from build123d import *

# Parameters (mm, degrees)
F0_R            = 304.8
F1_DEPTH        = 25.4
F2_DEPTH        = 25.4
F2_COPIES_COUNT = 31
F3_R            = 296.8625
F3_R_2          = 290.5125
F4_DEPTH        = 2.54
F5_R            = 296.8625
F5_R_2          = 290.5125
F6_DEPTH        = 2.54


# Not quite as in the source:
# - a pattern or mirror of a feature is missing from the dataset's text; its kind, count and spacing are read off the source's solid


with BuildPart() as f1:
    # F0 (on Top) → F1 (new body)
    with BuildSketch(Plane.XY):
        Circle(F0_R)
        with BuildLine():
            ThreePointArc((-139.9074929569, 241.8475830239), (139.5962149699, 242.0273884627), (279.4, 0))
            ThreePointArc((279.4, 0), (8.5793400064, -279.2682490457), (-278.873120437, -17.1505888444))
            Line((-278.873120437, -17.1505888444), (-284.48, -19.05))
            Line((-284.48, -19.05), (-284.48, 19.05))
            Line((-284.48, 19.05), (-278.873120437, 17.1505888444))
            ThreePointArc((-278.873120437, 17.1505888444), (-278.0539903617, 27.392306291), (-276.8588574341, 37.5969820635))
            Line((-276.8588574341, 37.5969820635), (-282.7052908844, 36.7727961626))
            Line((-282.7052908844, 36.7727961626), (-275.2642057328, 74.52500298))
            Line((-275.2642057328, 74.52500298), (-270.0959710932, 71.5019328355))
            ThreePointArc((-270.0959710932, 71.5019328355), (-267.303871456, 81.3203560288), (-264.1549850662, 91.0302359916))
            Line((-264.1549850662, 91.0302359916), (-270.1311147854, 91.3975495928))
            Line((-270.1311147854, 91.3975495928), (-255.2871620754, 126.8976403584))
            Line((-255.2871620754, 126.8976403584), (-250.8902083052, 122.9571607373))
            ThreePointArc((-250.8902083052, 122.9571607373), (-246.2317976323, 132.0388648646), (-241.2447866782, 140.9443610102))
            Line((-241.2447866782, 140.9443610102), (-247.0326592074, 142.4729997596))
            Line((-247.0326592074, 142.4729997596), (-225.5328396666, 174.384889715))
            Line((-225.5328396666, 174.384889715), (-221.9907783353, 169.6598194449))
            ThreePointArc((-221.9907783353, 169.6598194449), (-215.6401479473, 177.6617195494), (-209.0012374477, 185.4261112825))
            Line((-209.0012374477, 185.4261112825), (-214.453995901, 188.1291797331))
            Line((-214.453995901, 188.1291797331), (-187.0092810122, 215.058314286))
            Line((-187.0092810122, 215.058314286), (-184.5245635336, 209.7976297595))
            ThreePointArc((-184.5245635336, 209.7976297595), (-176.734130204, 216.4010333179), (-168.7075759898, 222.715320092))
            Line((-168.7075759898, 222.715320092), (-173.4326522734, 226.2997079893))
            Line((-173.4326522734, 226.2997079893), (-141.3964217588, 247.6183643131))
            Line((-141.3964217588, 247.6183643131), (-139.9074929569, 241.8475830239))
        make_face(mode=Mode.SUBTRACT)
        with BuildLine():
            ThreePointArc((-241.2447866782, 140.9443610102), (-232.0623656728, 155.6001877838), (-221.9907783353, 169.6598194449))
            Line((-221.9907783353, 169.6598194449), (-225.5328396666, 174.384889715))
            Line((-225.5328396666, 174.384889715), (-247.0326592074, 142.4729997596))
            Line((-247.0326592074, 142.4729997596), (-241.2447866782, 140.9443610102))
        make_face()
        with BuildLine():
            ThreePointArc((-209.0012374477, 185.4261112825), (-197.1398786083, 197.9904751807), (-184.5245635336, 209.7976297595))
            Line((-184.5245635336, 209.7976297595), (-187.0092810122, 215.058314286))
            Line((-187.0092810122, 215.058314286), (-214.453995901, 188.1291797331))
            Line((-214.453995901, 188.1291797331), (-209.0012374477, 185.4261112825))
        make_face()
        with BuildLine():
            ThreePointArc((-168.7075759898, 222.715320092), (-154.603771191, 232.7273811427), (-139.9074929569, 241.8475830239))
            Line((-139.9074929569, 241.8475830239), (-141.3964217588, 247.6183643131))
            Line((-141.3964217588, 247.6183643131), (-173.4326522734, 226.2997079893))
            Line((-173.4326522734, 226.2997079893), (-168.7075759898, 222.715320092))
        make_face()
        with BuildLine():
            Line((-270.1311147854, 91.3975495928), (-264.1549850662, 91.0302359916))
            ThreePointArc((-264.1549850662, 91.0302359916), (-258.0168985448, 107.1990674648), (-250.8902083052, 122.9571607373))
            Line((-250.8902083052, 122.9571607373), (-255.2871620754, 126.8976403584))
            Line((-255.2871620754, 126.8976403584), (-270.1311147854, 91.3975495928))
        make_face()
        with BuildLine():
            Line((-282.7052908844, 36.7727961626), (-276.8588574341, 37.5969820635))
            ThreePointArc((-276.8588574341, 37.5969820635), (-274.0023403806, 54.6541623845), (-270.0959710932, 71.5019328355))
            Line((-270.0959710932, 71.5019328355), (-275.2642057328, 74.52500298))
            Line((-275.2642057328, 74.52500298), (-282.7052908844, 36.7727961626))
        make_face()
        with BuildLine():
            Line((-284.48, -19.05), (-278.873120437, -17.1505888444))
            ThreePointArc((-278.873120437, -17.1505888444), (-279.4, 0), (-278.873120437, 17.1505888444))
            Line((-278.873120437, 17.1505888444), (-284.48, 19.05))
            Line((-284.48, 19.05), (-284.48, -19.05))
        make_face()
    extrude(amount=F1_DEPTH)

    # F0 (on Top) → F2 (join)
    with BuildSketch(Plane.XY):
        with BuildLine():
            ThreePointArc((-278.873120437, 17.1505888444), (-279.4, 0), (-278.873120437, -17.1505888444))
            Line((-278.873120437, -17.1505888444), (-256.3631135226, -9.525))
            ThreePointArc((-256.3631135226, -9.525), (-256.54, 0), (-256.3631135226, 9.525))
            Line((-256.3631135226, 9.525), (-278.873120437, 17.1505888444))
        make_face()
    f2 = extrude(amount=F2_DEPTH)

    # F2_copies: F2 ×31 about axis
    f2_copies_axis = Axis((0, 0, 0), (0, 0, 1))
    for i in range(1, F2_COPIES_COUNT):
        add(f2.rotate(f2_copies_axis, i * 360 / F2_COPIES_COUNT))

    # F3 (on face) → F4 (cut)
    with BuildSketch(Plane(origin=(0, 0, 0), x_dir=(1, 0, 0), z_dir=(0, 0, -1))):
        Circle(F3_R)
        Circle(F3_R_2, mode=Mode.SUBTRACT)
    extrude(amount=-F4_DEPTH, mode=Mode.SUBTRACT)

    # F5 (on face) → F6 (cut)
    with BuildSketch(Plane.XY.offset(25.4)):
        Circle(F5_R)
        Circle(F5_R_2, mode=Mode.SUBTRACT)
    extrude(amount=-F6_DEPTH, mode=Mode.SUBTRACT)


solid = f1.part
Work out the finished part from the listing and answer in its coordinate system (mm). A direction names the side the tool comes from. Coordinates: 2 decimals unless noted, no trailing zeros. Write each loop counter-clockwise with the first axis right and the second up, starting at its lowest first coordinate (ties: lowest second). Pieces come first, ordered by that corner, then holes. Notation, with made-up numbers: (48.25, -12) - (99.25, -12) arc R22 ccw to (99.25, 12) - close; hole circle Ø8 at (67, 17). An arc over 180 degrees is marked (long way). One line per question, with ' | ' between items.
1) Find section A-A, the plane y = 0. Determine the outline of the cut face in (x, z), and give its area (3 significant figures).
Checks:
outline: (-304.8, 0) - (-296.86, 0) - (-296.86, 2.54) - (-290.51, 2.54) - (-290.51, 0) - (-256.54, 0) - (-256.54, 25.4) - (-290.51, 25.4) - (-290.51, 22.86) - (-296.86, 22.86) - (-296.86, 25.4) - (-304.8, 25.4) - close; (279.4, 0) - (290.51, 0) - (290.51, 2.54) - (296.86, 2.54) - (296.86, 0) - (304.8, 0) - (304.8, 25.4) - (296.86, 25.4) - (296.86, 22.86) - (290.51, 22.86) - (290.51, 25.4) - (279.4, 25.4) - close | area: 1,810 mm2
2) Consider probe 1 along X at (y, z) = (273.5, 6); probe 2 along X at (y, z) = (96, 24.25); probe 3 along Y at (x, z) = (249, 12.5). Determine where each line is inside the solid, lowest interval first. Write a range as [from, to].
Checks:
probe 1: [-134.54, -26.12], [-1.34, 29.61], [53.35, 134.54] | probe 2: [-289.29, -280.91], [-274.19, -237.9], [255.68, 274.19], [280.91, 289.29] | probe 3: [-175.79, -119.77], [-91.12, -67.62], [67.62, 91.12], [119.77, 175.79]
3) Flat-ended cylindrical pins translate along their axes: P1, Ø3, axis at y = -154.5, z = 18, coming from the -X side; P2, Ø1, axis at y = -102.5, z = 12, coming from the -X side; P3, Ø10, axis at x = 201.5, z = 17, coming from the -Y side. Find the tip coordinate at first contact, or state that the pin passes through.
Checks:
P1: x = -263.62 | P2: x = -287.23 | P3: y = -233
4) For faces 1 (the face through (273, -124, 25.4)), 2 (the face through (197, -219, 22.86)), 3 (the face through (197, 219, 2.54)), 4 (the face through (54.18, -262.25, 12.52)), determine the directions among +Z, -Z, +X, -X, +Y, -Y from which every point of the face is accessible in a straight line to the end or side of a thin tool.
Checks:
face 1: +Z, +X, -X, +Y, -Y | face 2: +Z | face 3: -Z | face 4: +Z, -Z
5) The mould has two halves that part along Y. Classify faces 5 (the face through (-254, 54, 0)), 6 (the face through (-210.635, 146.444, 12.522)): +Y half, -Y half, draft (parallel to the pull), parting line (faces both ways), or undercut.
Checks:
face 5: draft | face 6: undercut
